Geometry check sheet. Reference: the model listing, model coordinates, mm. Face numbers are marked on the shaded views. Round coordinates to 2 decimals unless told otherwise and drop trailing zeros. Order: outer loops, then holes, each group sorted by start corner. A loop starts at its lowest first (then second) coordinate and runs counter-clockwise, first axis right, second up. Notation, with made-up numbers: (38.25, 60) - (71.25, 60) arc R23 ccw to (71.25, 68) - close; hole circle Ø8 at (-12.5, 8). An arc over 180 degrees is marked (long way). Use a Markdown table: item, result. Add a question column.
(1) Section check B-B on y = -12. Record the boundary of the cut face in (x, z), then the cut area to 3 significant figures.
(2) Mould release check, pull along Y, two halves, no side actions. Record for the marked faces 1, 2 and 3: released by +Y, released by -Y, zero draft, split by the parting line, or undercut.
(3) Section check A-A on z = 0. Record the boundary of the cut face in (x, y).
(4) Thickness scan on line 1 along Y through (x, z) = (5.5, -2.5); line 2 along Z through (x, y) = (2.5, 26); line 3 along Z through (x, y) = (5.25, 11.5). Record the ranges inside material, lowest first. Write a range as [from, to].
(5) Section check C-C on z = -11. Record the boundary of the cut face in (x, y), then the cut area to 3 significant figures.
(6) Gauge pin test, flat ends, axial feed: P1, Ø6, axis at x = 3.5, y = 4.5, coming from the -Z side (3 decimals); P2, Ø4, axis at x = 0.5, z = -23, coming from the +Y side; P3, Ø1, axis at x = 4, y = -13, coming from the +Z side. Record the tip position at first contact, or that the pin passes through.
Autodesk Inventor part; units mm, degrees
ref_plane "YZ Plane" through (0, 0, 0) normal (1, 0, 0) x (0, 1, 0)
ref_plane "XZ Plane" through (0, 0, 0) normal (0, 1, 0) x (-1, 0, 0)
ref_plane "XY Plane" through (0, 0, 0) normal (0, 0, 1) x (1, 0, 0)
sketch "スケッチ1" plane through (0, 0, 0) normal (1, 0, 0) x (0, 1, 0)
  circle A0 centre (0, 0) radius 45
  dimension "d0" = 90
extrude "押し出し1" add sketch "スケッチ1" along normal blind 10
sketch "スケッチ2" plane through (10, 0, 0) normal (1, 0, 0) x (0, 0, -1)
  circle A0 centre (0, 0) radius 46
  dimension "d3" = 92
extrude "押し出し2" add sketch "スケッチ2" along normal blind 1
sketch "スケッチ3" plane through (0, 0, 0) normal (-1, 0, 0) x (0, 0, 1)
  circle A0 centre (0, 0.7888) radius 46
  point P0 (0, 0)
  dimension "d6" = 92
extrude "押し出し3" add sketch "スケッチ3" along normal blind 1
sketch "スケッチ4" plane through (-1, 0.7888, 0) normal (-1, 0, 0) x (0, 0, 1)
  point P0 (0, -0.7888)
sketch "スケッチ5" plane through (-1, 0.7888, 0) normal (-1, 0, 0) x (0, 0, 1)
  circle A0 centre (0, 0) radius 6
  circle A1 centre (0, 0) radius 46
  point P0 (0, -0.7888)
  dimension "d9" = 12
  dimension "d10" = 40
extrude "押し出し4" cut sketch "スケッチ5" against normal blind 12 contours A0
equation "\"BendRadius\" = Thickness"
equation "\"BendReliefWidth\" = Thickness"
equation "\"BendReliefDepth\" = 0.5 * Thickness"
equation "\"CornerReliefSize\" = 4 * Thickness"
equation "\"MinimumRemnant\" = 2 * Thickness"
equation "\"TransitionRadius\" = BendRadius"
equation "\"JacobiRadiusSize\" = BendRadius"
equation "\"GapSize\" = Thickness"
properties part number "type3" material "アセタール樹脂、白"
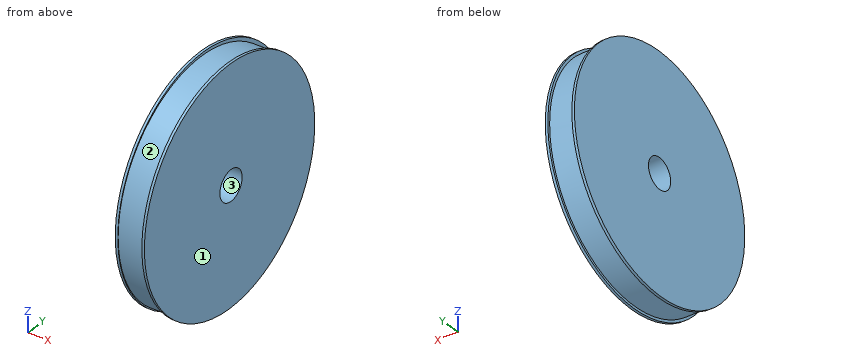
Check sheet entries:
| question | item | result |
|---|---|---|
| 1 | outline | (-1, -44.19) - (0, -44.19) - (0, -43.37) - (10, -43.37) - (10, -44.41) - (11, -44.41) - (11, 44.41) - (10, 44.41) - (10, 43.37) - (0, 43.37) - (0, 44.19) - (-1, 44.19) - close |
| 1 | area | 1,040 mm2 |
| 2 | face 1 | zero draft |
| 2 | face 2 | split by the parting line |
| 2 | face 3 | undercut |
| 3 | outline | (-1, -45.21) - (0, -45.21) - (0, -45) - (10, -45) - (10, -46) - (11, -46) - (11, -5.21) - (-1, -5.21) - close; (-1, 6.79) - (11, 6.79) - (11, 46) - (10, 46) - (10, 45) - (0, 45) - (0, 46.79) - (-1, 46.79) - close |
| 4 | line 1 | y = [-44.93, -4.67], [6.24, 44.93] |
| 4 | line 2 | z = [-36.73, 36.73] |
| 4 | line 3 | z = [-43.51, 43.51] |
| 5 | outline | (-1, -43.88) - (0, -43.88) - (0, -43.63) - (10, -43.63) - (10, -44.67) - (11, -44.67) - (11, 44.67) - (10, 44.67) - (10, 43.63) - (0, 43.63) - (0, 45.45) - (-1, 45.45) - close |
| 5 | area | 1,050 mm2 |
| 6 | P1 | stops at z = -44.975 |
| 6 | P2 | stops at y = 41.68 |
| 6 | P3 | stops at z = 43.23 |
